For this review, take the finished solid that the model builds, in its own axes (mm). Face numbers are marked on the shaded views. A direction names the side the tool comes from. Coordinates: 2 decimals unless noted, no trailing zeros. Order: outer loops, then holes, each group sorted by start corner. A loop starts at its lowest first (then second) coordinate and runs counter-clockwise, first axis right, second up.
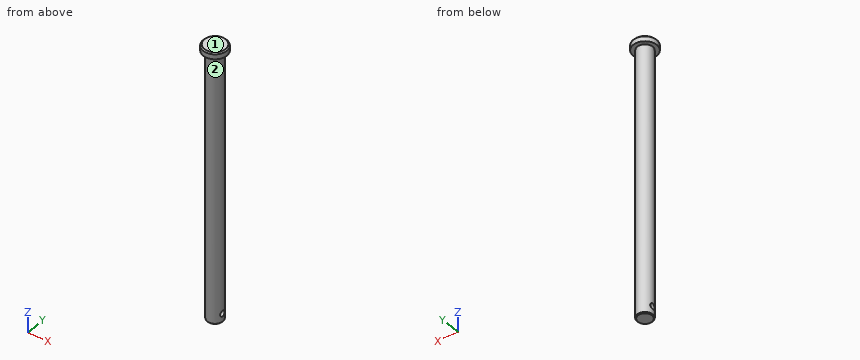
from build123d import *

# Parameters (mm, degrees)
SKETCH1_R           = 3.175
EXTRUDE1_DEPTH      = 55
SKETCH2_R           = 4.826
EXTRUDE2_DEPTH      = 2.54
CHAMFER1_SIZE       = 0.508
EXTRUDE3_DEPTH      = 58.943352958
EXTRUDE3_DEPTH_BACK = 58.943352958
SKETCH3_R           = 1.190625
CHAMFER2_SIZE       = 0.3175


with BuildPart() as part:
    # Sketch1 → Extrude1 (new, symmetric)
    with BuildSketch(Plane.XY):
        Circle(SKETCH1_R)
    extrude(amount=EXTRUDE1_DEPTH, both=True)

    # Sketch2 → Extrude2 (add)
    with BuildSketch(Plane.XY.offset(55)):
        Circle(SKETCH2_R)
    extrude(amount=EXTRUDE2_DEPTH)

    # Chamfer1
    chamfer1_edges = [part.edges().sort_by_distance(p)[0] for p in [
        (-4.826, 0, 57.54),
    ]]
    chamfer(chamfer1_edges, length=CHAMFER1_SIZE)

    # Sketch3 → Extrude3 (cut, two sides: drawn at the far end of the back side and taken through both)
    with BuildSketch(Plane(origin=(0, 0, 0), x_dir=(0, 0, -1), z_dir=(1, 0, 0)).offset(-EXTRUDE3_DEPTH_BACK)):
        with Locations(Location((51.42495, 0, 0), (0, 0, 179.999999999))):
            Circle(SKETCH3_R)
    extrude(amount=EXTRUDE3_DEPTH + EXTRUDE3_DEPTH_BACK, mode=Mode.SUBTRACT)

    # Chamfer2
    chamfer2_edges = [part.edges().sort_by_distance(p)[0] for p in [
        (-3.175, 0, -55),
    ]]
    chamfer(chamfer2_edges, length=CHAMFER2_SIZE)


solid = part.part
1. Take a section at B-B, the plane x = 0. Give the boundary of the cut face in (y, z) (1 decimal).
Answer below:
outline: (-4.8, 55) - (-3.2, 55) - (-3.2, -54.7) - (-2.9, -55) - (2.9, -55) - (3.2, -54.7) - (3.2, 55) - (4.8, 55) - (4.8, 57) - (4.3, 57.5) - (-4.3, 57.5) - (-4.8, 57) - close; hole circle Ø2.4 at (0, -51.4)
2. Take a section at C-C, the plane z = -16. Give the boundary of the cut face in (x, y) (3 decimals).
Answer below:
outline: circle Ø6.35 at (0, 0)
3. Machinability: for the marked faces 1 and 2, which of the approach directions +Z, -Z, +X, -X, +Y, -Y give a long, thin tool a straight path to every point of the face, cutting with its end or side? Answer none if there is none.
Answer below:
face 1: +Z, +X, -X, +Y, -Y
face 2: -Z
4. To check wall thickness, follow L1, parallel to Z at x = 1.75, y = 0.5; L2, parallel to Z at x = 2.5, y = -3; L3, parallel to Z at x = 0.5, y = -0.25. State the ranges of each line that lie inside material, in increasing order.
Answer below:
L1: z = -55 to -52.51, -50.34 to 57.54
L2: z = 55 to 57.54
L3: z = -55 to -52.59, -50.26 to 57.54
5. Clearance check with flat-ended pins moving along their axes: pin 1 Ø2 at (x, z) = (3, 15) entering from +Y; pin 2 Ø3 at (y, z) = (0, -51.42) entering from -X (3 decimals); pin 3 Ø5 at (y, z) = (-3, 38) entering from +X. State where each tip first meets the part, or that it passes through.
Answer below:
pin 1: stops at y = 2.47
pin 2: stops at x = -3.175
pin 3: stops at x = 3.14
6. Take a section at A-A, the plane y = 0. Give the boundary of the cut face in (x, z) (1 decimal).
Answer below:
outline: (-4.8, 55) - (-3.2, 55) - (-3.2, -50.2) - (3.2, -50.2) - (3.2, 55) - (4.8, 55) - (4.8, 57) - (4.3, 57.5) - (-4.3, 57.5) - (-4.8, 57) - close; (-3.2, -54.7) - (-2.9, -55) - (2.9, -55) - (3.2, -54.7) - (3.2, -52.6) - (-3.2, -52.6) - close
